from build123d import *

# Parameters (mm, degrees)
SKETCH2_W           = 80
SKETCH2_H           = 60
BOSS_EXTRUDE1_DEPTH = 3
SKETCH3_W           = 15
SKETCH3_H           = 25
CUT_EXTRUDE1_DEPTH  = 1
SKETCH4_R           = 1
CUT_EXTRUDE3_DEPTH  = 2
FILLET1_R           = 5
SKETCH5_R           = 1
CUT_EXTRUDE4_DEPTH  = 3
SKETCH6_W           = 15
SKETCH6_H           = 25
CUT_EXTRUDE6_DEPTH  = 1
SKETCH7_R           = 1
CUT_EXTRUDE7_DEPTH  = 7


with BuildPart() as part:
    # Sketch2 → Boss-Extrude1 (new body)
    with BuildSketch(Plane(origin=(0, 0, 0), x_dir=(1, 0, 0), z_dir=(0, 1, 0))):
        with Locations((-19.25, -4.5)):
            Rectangle(SKETCH2_W, SKETCH2_H)
    extrude(amount=BOSS_EXTRUDE1_DEPTH)

    # Sketch3 → Cut-Extrude1 (cut)
    with BuildSketch(Plane.XZ):
        with Locations((-51.75, 4.5)):
            Rectangle(SKETCH3_W, SKETCH3_H)
    extrude(amount=-CUT_EXTRUDE1_DEPTH, mode=Mode.SUBTRACT)

    # Sketch4 → Cut-Extrude3 (cut)
    with BuildSketch(Plane.XZ.offset(-1)):
        with Locations(Location((-51.75, 12.5, 0), (0, 0, 270))):
            Circle(SKETCH4_R)
        with Locations(Location((-51.75, -3.5, 0), (0, 0, 270))):
            Circle(SKETCH4_R)
    extrude(amount=-CUT_EXTRUDE3_DEPTH, mode=Mode.SUBTRACT)

    # Fillet1
    fillet1_edges = [part.edges().sort_by_distance(p)[0] for p in [
        (-59.25, 1.5, -25.5),
        (20.75, 1.5, -25.5),
        (20.75, 1.5, 34.5),
        (-59.25, 1.5, 34.5),
    ]]
    fillet(fillet1_edges, radius=FILLET1_R)

    # Sketch5 → Cut-Extrude4 (cut)
    with BuildSketch(Plane.XZ):
        with Locations(Location((-19.25, 4.5, 0), (0, 0, 270))):
            Circle(SKETCH5_R)
    extrude(amount=-CUT_EXTRUDE4_DEPTH, mode=Mode.SUBTRACT)

    # Sketch6 → Cut-Extrude6 (cut)
    with BuildSketch(Plane(origin=(0, 0, 0), x_dir=(1, 0, 0), z_dir=(0, 1, 0))):
        with Locations((13.25, -4.5)):
            Rectangle(SKETCH6_W, SKETCH6_H)
    extrude(amount=CUT_EXTRUDE6_DEPTH, mode=Mode.SUBTRACT)

    # Sketch7 → Cut-Extrude7 (cut)
    with BuildSketch(Plane(origin=(0, 0, 0), x_dir=(1, 0, 0), z_dir=(0, 1, 0))):
        with Locations(Location((13.25, 3.5, 0), (0, 0, 90))):
            Circle(SKETCH7_R)
        with Locations(Location((13.25, -12.5, 0), (0, 0, 90))):
            Circle(SKETCH7_R)
    extrude(amount=CUT_EXTRUDE7_DEPTH, mode=Mode.SUBTRACT)


solid = part.part
Source: CAD feature listing. Evaluate the final solid. Frame: model axes, mm. A direction names the side the tool comes from. Round coordinates to 2 decimals unless told otherwise and drop trailing zeros. Loops run counter-clockwise (first coordinate to the right, second up) from the corner with the lowest first, then second, coordinate; pieces in that order, holes last. Notation, with made-up numbers: (34, 68) - (91, 68) arc R18 cw to (91, 85) - close; hole circle Ø1 at (-38.75, -9). An arc over 180 degrees is marked (long way). Write item = value, one per line. Start each with the question number.
Item 1: Section query D-D on z = -3.5. Output: boundary loops of the cut face in (x, y), plus the area to 3 significant figures.
Item 2: Mould query, pull axis Z, two halves, no side actions, for faces 4 (the face through (14.226, 1.986, 12.717)), 5 (the face through (-59.25, 2, 5)), 6 (the face through (-20, 1, 34.5)). Classes: released by +Z, released by -Z, zero draft, split by the parting line, or undercut.
Item 3: Section query B-B on z = 4.5. Output: boundary loops of the cut face in (x, y), plus the area to 3 significant figures.
Item 4: Reachability of faces 1 (the face through (-57.82, 1.52, 33)), 2 (the face through (-52, 1, 5)), 3 (the face through (13, 1, 4)) from +Z, -Z, +X, -X, +Y, -Y: full face, straight path, thin tool, end or side. Return the list, or none.
Item 5: First-contact query: pin 1 Ø3 at (x, z) = (-51.75, -3.5) entering from +Y; pin 2 Ø2.5 at (x, z) = (13.25, 12.5) entering from -Y; pin 3 Ø0.5 at (y, z) = (0.5, 9) entering from -X; pin 4 Ø0.8 at (y, z) = (0.5, 1.5) entering from +X. Flat tips, straight axial feed; report the tip coordinate or a pass-through.
Item 6: Material intervals for line 1 (X direction, y = 2.4, z = 12.5); line 2 (Z direction, x = -54.5, y = 0.95); line 3 (X direction, y = 1.6, z = 4.5), sorted ascending.
Item 7: Section query C-C on x = 13.25. Output: boundary loops of the cut face in (y, z), plus the area to 3 significant figures.
Item 8: Section query A-A on x = -19.25. Output: boundary loops of the cut face in (y, z).
Results list:
q1.outline = (-59.25, 1) - (-52.75, 1) - (-52.75, 3) - (-59.25, 3) - close; (-50.75, 1) - (-44.25, 1) - (-44.25, 0) - (5.75, 0) - (5.75, 1) - (12.25, 1) - (12.25, 3) - (-50.75, 3) - close; (14.25, 1) - (20.75, 1) - (20.75, 3) - (14.25, 3) - close
q1.area = 202 mm²
q2.face_4 = undercut
q2.face_5 = zero draft
q2.face_6 = released by +Z
q3.outline = (-59.25, 1) - (-44.25, 1) - (-44.25, 0) - (-20.25, 0) - (-20.25, 3) - (-59.25, 3) - close; (-18.25, 0) - (5.75, 0) - (5.75, 1) - (20.75, 1) - (20.75, 3) - (-18.25, 3) - close
q3.area = 204 mm²
q4.face_1 = +Z, -X, +Y, -Y
q4.face_2 = -X, -Y
q4.face_3 = +X, -Y
q5.pin_1 = 3
q5.pin_2 = 1
q5.pin_3 = -44.25
q5.pin_4 = 5.75
q6.line_1 = -59.25 to -52.75, -50.75 to 12.25, 14.25 to 20.75
q6.line_2 = -25.49 to -8, 17 to 34.49
q6.line_3 = -59.25 to -20.25, -18.25 to 20.75
q7.outline = (0, -25.5) - (3, -25.5) - (3, -4.5) - (1, -4.5) - (1, -8) - (0, -8) - close; (0, 17) - (1, 17) - (1, 13.5) - (3, 13.5) - (3, 34.5) - (0, 34.5) - close; (1, -2.5) - (3, -2.5) - (3, 11.5) - (1, 11.5) - close
q7.area = 147 mm²
q8.outline = (0, -25.5) - (3, -25.5) - (3, 3.5) - (0, 3.5) - close; (0, 5.5) - (3, 5.5) - (3, 34.5) - (0, 34.5) - close
